Job drawing, mm, ordinate dimensions from the low corner. One solid piece. A direction names the side the tool comes from. Give positions to 0.01 mm unless a question says otherwise; leave off trailing zeros. Loops run counter-clockwise (first coordinate to the right, second up) from the corner with the lowest first, then second, coordinate; pieces in that order, holes last. Notation, with made-up numbers: (-37, -40) - (6, -40) arc R19 cw to (6, -6) - close; hole circle Ø9 at (65, -6.75). An arc over 180 degrees is marked (long way). Use a Markdown table: item, result.
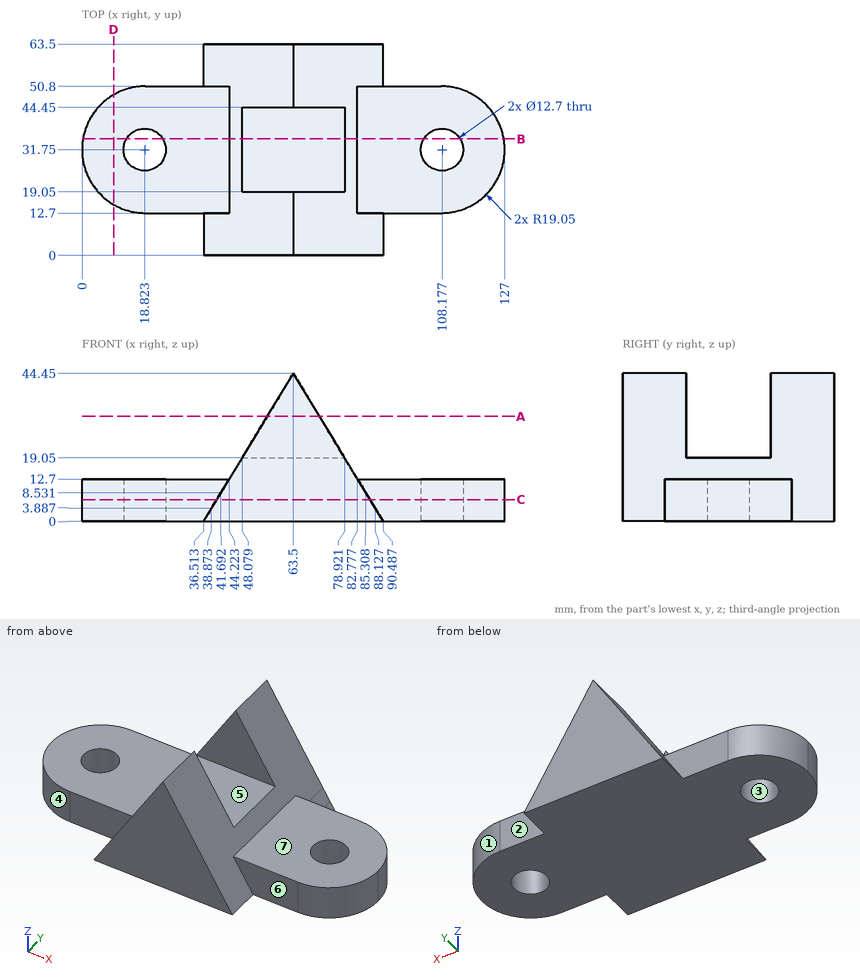
(1) Slice it at B-B, the plane y = 35. Write the cut outline in (x, z), plus the area to 3 significant figures.
Computed:
| item | result |
|---|---|
| outline | (0.28, 0) - (13.37, 0) - (13.37, 12.7) - (0.28, 12.7) - close; (24.28, 0) - (102.72, 0) - (102.72, 12.7) - (82.78, 12.7) - (78.92, 19.05) - (48.08, 19.05) - (44.22, 12.7) - (24.28, 12.7) - close; (113.63, 0) - (126.72, 0) - (126.72, 12.7) - (113.63, 12.7) - close |
| area | 1,550 mm² |
(2) Pin check, flat tips, straight feed: P1, Ø10, axis at x = 18.82, y = 31.75, coming from the +Z side; P2, Ø11.5, axis at x = 26, y = 35.5, coming from the +Z side; P3, Ø12, axis at x = 63.5, y = 27.5, coming from the +Z side; P4, Ø6.5, axis at x = 31.5, z = 8, coming from the +Y side. Stop position of each tip, or through.
Computed:
| item | result |
|---|---|
| P1 | through |
| P2 | z = 12.7 |
| P3 | z = 19.05 |
| P4 | y = 50.8 |
(3) Mould opens along X. For the marked faces 1, 2, 3 and 4 say: pulls with the +X half, pulls with the -X half, needs draft (parallel to the pull), parting line crosses it, or undercut.
Computed:
| item | result |
|---|---|
| face 1 | pulls with the +X half |
| face 2 | needs draft |
| face 3 | undercut |
| face 4 | pulls with the -X half |
(4) Slice it at D-D, the plane x = 9.5. Write the cut outline in (y, z).
Computed:
| item | result |
|---|---|
| outline | (15.27, 0) - (48.23, 0) - (48.23, 12.7) - (15.27, 12.7) - close |
(5) Slice it at C-C, the plane z = 6.5. Count the separate pieces of the cut face and the enclosed holes in it, plus the area to 3 significant figures.
Computed:
| item | result |
|---|---|
| separate pieces | 1 |
| enclosed holes | 2 |
| area | 5,440 mm² |
(6) 3-axis set-ups, long thin cutter, end or side, ignore diameter. For the marked faces 5, 6 and 7: which of +Z, -Z, +X, -X, +Y, -Y reach the whole face in a straight line?
Computed:
| item | result |
|---|---|
| face 5 | +Z, +X, -X |
| face 6 | +Z, +X, -Y |
| face 7 | +Z, +X, +Y, -Y |
(7) Slice it at A-A, the plane z = 31.5. Write the cut outline in (x, y).
Computed:
| item | result |
|---|---|
| outline | (55.64, 0) - (71.36, 0) - (71.36, 19.05) - (55.64, 19.05) - close; (55.64, 44.45) - (71.36, 44.45) - (71.36, 63.5) - (55.64, 63.5) - close |
(8) Drill centre lines: probe 1 along Y at (x, z) = (66, 21.5); probe 2 along X at (y, z) = (31, 3) (1 decimal); probe 3 along X at (y, z) = (27, 9) (1 decimal). Where is each one in solid material? Low to high. Write a range as [from, to].
Computed:
| item | result |
|---|---|
| probe 1 | [0, 19.05], [44.45, 63.5] |
| probe 2 | [0, 12.5], [25.1, 101.9], [114.5, 127] |
| probe 3 | [0.6, 14.6], [23, 104], [112.4, 126.4] |
